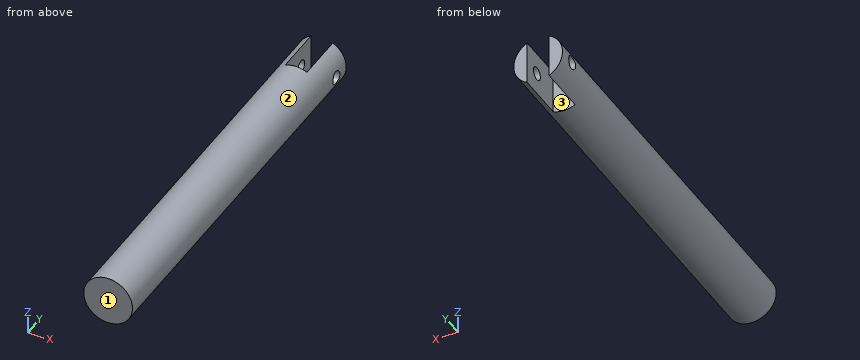
from build123d import *

# Parameters (mm, degrees)
SKETCH1_R               = 10
BOSS_EXTRUDE1_DEPTH     = 165
CUT_EXTRUDE1_DEPTH      = 166.604951617
CUT_EXTRUDE1_DEPTH_BACK = 166.604951617
SKETCH2_W               = 9
SKETCH2_H               = 40
CUT_EXTRUDE2_DEPTH      = 166.604951617
CUT_EXTRUDE2_DEPTH_BACK = 166.604951617
SKETCH3_R               = 2.7


with BuildPart() as part:
    # Sketch1 → Boss-Extrude1 (new body)
    with BuildSketch(Plane(origin=(0, 0, 0), x_dir=(1, 0, 0), z_dir=(0, 1, 0))):
        with Locations(Location((0, 0, 0), (0, 0, 270))):
            Circle(SKETCH1_R)
    extrude(amount=BOSS_EXTRUDE1_DEPTH)

    # Sketch2 → Cut-Extrude1 (cut, two sides: drawn at the far end of the back side and taken through both)
    with BuildSketch(Plane.XY.offset(-CUT_EXTRUDE1_DEPTH_BACK)):
        with Locations((0, 165)):
            Rectangle(SKETCH2_W, SKETCH2_H)
    extrude(amount=CUT_EXTRUDE1_DEPTH + CUT_EXTRUDE1_DEPTH_BACK, mode=Mode.SUBTRACT)

    # Sketch3 → Cut-Extrude2 (cut, two sides: drawn at the far end of the back side and taken through both)
    with BuildSketch(Plane(origin=(0, 0, 0), x_dir=(0, 0, -1), z_dir=(1, 0, 0)).offset(-CUT_EXTRUDE2_DEPTH_BACK)):
        with Locations(Location((0, 157.5, 0), (0, 0, 270))):
            Circle(SKETCH3_R)
    extrude(amount=CUT_EXTRUDE2_DEPTH + CUT_EXTRUDE2_DEPTH_BACK, mode=Mode.SUBTRACT)


solid = part.part
Can you work these out from the model? Positions are in its coordinate system, mm. Face numbers are marked on the shaded views. Give positions to 0.01 mm unless a question says otherwise; leave off trailing zeros. Order: outer loops, then holes, each group sorted by start corner. A loop starts at its lowest first (then second) coordinate and runs counter-clockwise, first axis right, second up. Notation, with made-up numbers: (35.25, -37.5) - (75.25, -37.5) arc R30 cw to (75.25, -11.5) - close; hole circle Ø9 at (2.5, -13). An arc over 180 degrees is marked (long way). Write each question's results on one line, items separated by ' | '.
1) Suppose I cut it at B-B, the plane z = 0. Write out the boundary of the cut face in (x, y), then the cut area to 3 significant figures.
Final values:
outline: (-10, 0) - (10, 0) - (10, 154.8) - (4.5, 154.8) - (4.5, 145) - (-4.5, 145) - (-4.5, 154.8) - (-10, 154.8) - close; (-10, 160.2) - (-4.5, 160.2) - (-4.5, 165) - (-10, 165) - close; (4.5, 160.2) - (10, 160.2) - (10, 165) - (4.5, 165) - close | area: 3,060 mm^2
2) Suppose I cut it at D-D, the plane z = -7. Write out the boundary of the cut face in (x, y).
Final values:
outline: (-7.14, 0) - (7.14, 0) - (7.14, 165) - (4.5, 165) - (4.5, 145) - (-4.5, 145) - (-4.5, 165) - (-7.14, 165) - close
3) Suppose I cut it at A-A, the plane y = 157.5. Write out the boundary of the cut face in (x, z).
Final values:
outline: (-9.63, -2.7) arc R10 ccw to (-4.5, -8.93) - (-4.5, -2.7) - close; (-9.63, 2.7) - (-4.5, 2.7) - (-4.5, 8.93) arc R10 ccw to start; (4.5, -8.93) arc R10 ccw to (9.63, -2.7) - (4.5, -2.7) - close; (4.5, 2.7) - (9.63, 2.7) arc R10 ccw to (4.5, 8.93) - close
4) If we mould it in two halves opening along X, with no side actions, what happens to the marked faces 1, 2 and 3? For each: pulls with the +X half, pulls with the -X half, needs draft (parallel to the pull), parting line crosses it, or undercut.
Final values:
face 1: needs draft | face 2: parting line crosses it | face 3: undercut
5) Please list where these lines run through material, in increasing order: line 1 along Z through (x, y) = (-0.75, 49); line 2 along Y through (x, z) = (4.25, -3.25); line 3 along Z through (x, y) = (-5.9, 157.5). Write a range as [from, to].
Final values:
line 1: z = [-9.97, 9.97] | line 2: y = [0, 145] | line 3: z = [-8.07, -2.7], [2.7, 8.07]
6) I'm going to push flat-ended pins straight in: pin 1 Ø4.5 at (x, z) = (-1.5, -0.5) entering from +Y; pin 2 Ø5.5 at (y, z) = (156.5, 0.5) entering from -X; pin 3 Ø3 at (x, y) = (-4, 136) entering from +Z; pin 4 Ø8 at (x, y) = (-4.5, 39) entering from -Z. Where does each tip first touch, or does it pass through?
Final values:
pin 1: stops at y = 145 | pin 2: stops at x = -10 | pin 3: stops at z = 9.68 | pin 4: stops at z = -9.99
7) Suppose I cut it at C-C, the plane x = 6.25. Write out the boundary of the cut face in (y, z), then the cut area to 3 significant figures.
Final values:
outline: (0, -7.81) - (165, -7.81) - (165, 7.81) - (0, 7.81) - close; hole circle Ø5.4 at (157.5, 0) | area: 2,550 mm^2
